Print and shaded views of the part. All mm, measured from the part's lowest x, y and z. Give positions to 0.01 mm unless a question says otherwise; leave off trailing zeros. Loops run counter-clockwise (first coordinate to the right, second up) from the corner with the lowest first, then second, coordinate; pieces in that order, holes last. Notation, with made-up numbers: M 32,-8 L 85,-8 A9 cw 85,-1 Z; hole C 76.5,0 d4. An arc over 180 degrees is marked long. Answer as CSV lines item,"result".
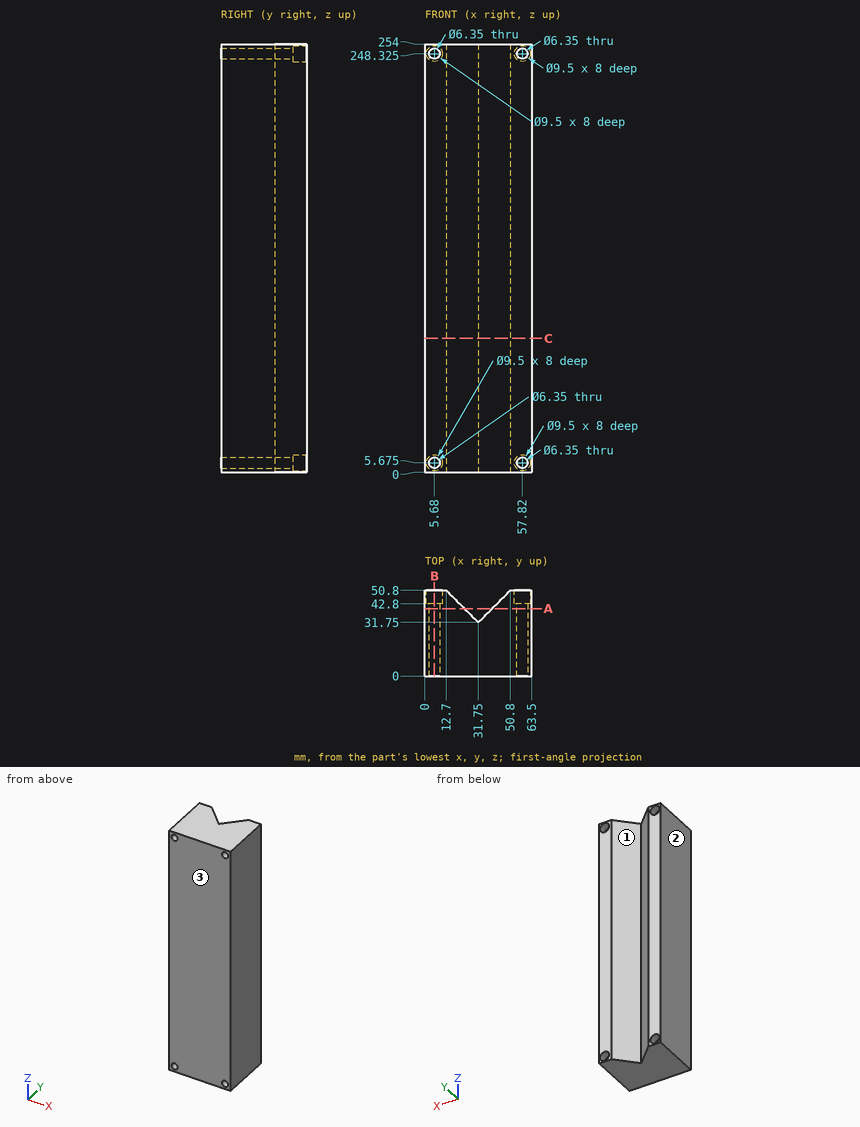
Q1. Cut at A-A (y = 40). Write the cut outline in (x, z) (3 decimals).
Solution:
outline,"M 0,0 L 23.5,0 L 23.5,254 L 0,254 Z; M 40,0 L 63.5,0 L 63.5,254 L 40,254 Z; hole C 5.68,5.675 d6.35; hole C 5.68,248.325 d6.35; hole C 57.82,5.675 d6.35; hole C 57.82,248.325 d6.35"
Q2. Cut at C-C (z = 79.5). Write the cut outline in (x, y).
Solution:
outline,"M 0,0 L 63.5,0 L 63.5,50.8 L 50.8,50.8 L 31.75,31.75 L 12.7,50.8 L 0,50.8 Z"
Q3. Cut at B-B (x = 5.68). Write the cut outline in (y, z) (3 decimals).
Solution:
outline,"M 0,0 L 50.8,0 L 50.8,0.925 L 42.8,0.925 L 42.8,2.5 L 0,2.5 Z; M 0,8.85 L 42.8,8.85 L 42.8,10.425 L 50.8,10.425 L 50.8,243.575 L 42.8,243.575 L 42.8,245.15 L 0,245.15 Z; M 0,251.5 L 42.8,251.5 L 42.8,253.075 L 50.8,253.075 L 50.8,254 L 0,254 Z"
Q4. Pin check, flat tips, straight feed: P1, Ø7.5, axis at x = 57.82, z = 5.675, coming from the +Y side; P2, Ø3, axis at x = 6, z = 248.5, coming from the +Y side; P3, Ø5, axis at x = 33.5, z = 129, coming from the +Y side. Stop position of each tip, or through.
Solution:
P1,"stops at y = 42.8"
P2,"passes through"
P3,"stops at y = 36"
Q5. Wall check: line 1 (Z direction, x = 5, y = 49); line 2 (Z direction, x = 58, y = 29.5); line 3 (X direction, y = 33.5, z = 147.5). Give the ranges that are in metal, low to high. Write a range as [from, to].
Solution:
line 1,"z = [0, 0.97], [10.38, 243.62], [253.03, 254]"
line 2,"z = [0, 2.51], [8.84, 245.16], [251.49, 254]"
line 3,"x = [0, 30], [33.5, 63.5]"
Q6. Mould opens along X. For the marked faces 1, 2 and 3 say: released by +X, released by -X, zero draft, split by the parting line, or undercut.
Solution:
face 1,"undercut"
face 2,"released by -X"
face 3,"zero draft"
